Answer from the drawing. Dimensions are ordinates in mm from the lowest x, y and z of the part. A direction names the side the tool comes from. Coordinates: 2 decimals unless noted, no trailing zeros. Write each loop counter-clockwise with the first axis right and the second up, starting at its lowest first coordinate (ties: lowest second). Pieces come first, ordered by that corner, then holes. Notation, with made-up numbers: (-32, -40) - (3, -40) arc R18 cw to (3, -27) - close; hole circle Ø1 at (-34, 49). An arc over 180 degrees is marked (long way). Use a Markdown table: item, result.
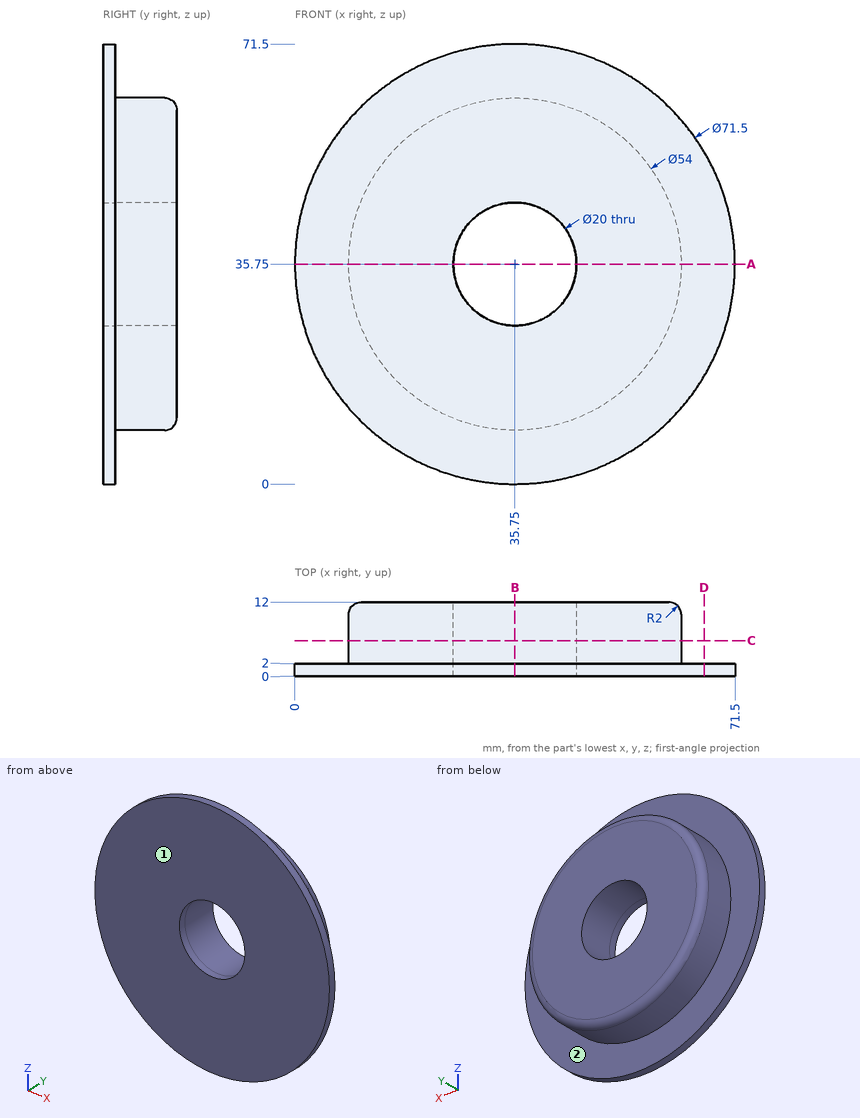
(1) Straight lines are drawn through the part: L1, parallel to Z at x = 35.75, y = 8.5; L2, parallel to Z at x = 35.75, y = 1.5; L3, parallel to Y at x = 20, z = 67. For each, find the intervals that lie inside material, in ascending order.
Report:
| item | result |
|---|---|
| L1 | z = 8.75 to 25.75, 45.75 to 62.75 |
| L2 | z = 0 to 25.75, 45.75 to 71.5 |
| L3 | y = 0 to 2 |
(2) A cutting plane is placed at C-C, the plane y = 5.75. Write down the section's boundary in (x, z), and give its area (3 significant figures).
Report:
| item | result |
|---|---|
| outline | circle Ø54 at (35.75, 35.75); hole circle Ø20 at (35.75, 35.75) |
| area | 1,980 mm² |
(3) For the marked faces 1 and 2, determine the directions among +Z, -Z, +X, -X, +Y, -Y from which every point of the face is accessible in a straight line to the end or side of a thin tool.
Report:
| item | result |
|---|---|
| face 1 | +Z, -Z, +X, -X, -Y |
| face 2 | +Y |
(4) A cutting plane is placed at B-B, the plane x = 35.75. Write down the section's boundary in (y, z), and give its area (3 significant figures).
Report:
| item | result |
|---|---|
| outline | (0, 0) - (2, 0) - (2, 8.75) - (10, 8.75) arc R2 ccw to (12, 10.75) - (12, 25.75) - (0, 25.75) - close; (0, 45.75) - (12, 45.75) - (12, 60.75) arc R2 ccw to (10, 62.75) - (2, 62.75) - (2, 71.5) - (0, 71.5) - close |
| area | 441 mm² |
(5) A cutting plane is placed at A-A, the plane z = 35.75. Write down the section's boundary in (x, y).
Report:
| item | result |
|---|---|
| outline | (0, 0) - (25.75, 0) - (25.75, 12) - (10.75, 12) arc R2 ccw to (8.75, 10) - (8.75, 2) - (0, 2) - close; (45.75, 0) - (71.5, 0) - (71.5, 2) - (62.75, 2) - (62.75, 10) arc R2 ccw to (60.75, 12) - (45.75, 12) - close |
(6) A cutting plane is placed at D-D, the plane x = 66.5. Write down the section's boundary in (y, z), and give its area (3 significant figures).
Report:
| item | result |
|---|---|
| outline | (0, 17.52) - (2, 17.52) - (2, 53.98) - (0, 53.98) - close |
| area | 72.9 mm² |
(7) Each of these flat-tipped pins is pushed along its axis until it touches: P1, Ø6, axis at x = 11.5, z = 20.5, coming from the +Y side; P2, Ø4, axis at x = 53.5, y = 7.5, coming from the -Z side; P3, Ø4, axis at y = 9.5, z = 44.5, coming from the +X side. Where does it stop, or does it pass through?
Report:
| item | result |
|---|---|
| P1 | stops at y = 11.89 |
| P2 | stops at z = 13.82 |
| P3 | stops at x = 61.89 |
